Could you check a few things on this model? Use its own coordinates, in mm. Face numbers are marked on the shaded views. Coordinates: 2 decimals unless noted, no trailing zeros. Write each loop counter-clockwise with the first axis right and the second up, starting at its lowest first coordinate (ties: lowest second). Pieces come first, ordered by that corner, then holes. Notation, with made-up numbers: (-3, 67) - (51, 67) arc R19 ccw to (51, 84) - close; hole circle Ø5 at (35.5, 40.5). An arc over 180 degrees is marked (long way). Answer as a JSON object with one key per item and string values. Group by question number.
1) If we section it at B-B (y = -70): Write out the boundary of the cut face in (x, z).
2) If we section it at D-D (x = 70): Write out the boundary of the cut face in (y, z).
3) We'd pull the mould along Y, two halves only. Please class the marked faces 1, 2, 3 and 4: released by +Y, released by -Y, zero draft, split by the parting line, or undercut.
4) If we section it at A-A (y = -30): Write out the boundary of the cut face in (x, z).
5) Will these pins go through, and if not, where does the flat tip stop? pin 1 Ø5 at (x, y) = (30, -30) entering from -Z; pin 2 Ø2.5 at (x, z) = (22, 9.5) entering from -Y; pin 3 Ø4 at (y, z) = (-14.5, 9) entering from +X; pin 4 Ø24 at (x, y) = (38, -52.5) entering from +Z.
6) Please list where these lines run through material, in increasing order: line 1 along X through (y, z) = (-13, 10); line 2 along Y through (x, z) = (30, 1.85); line 3 along X through (y, z) = (-51, 3).
7) If we section it at C-C (z = 10): Write out the boundary of the cut face in (x, y).
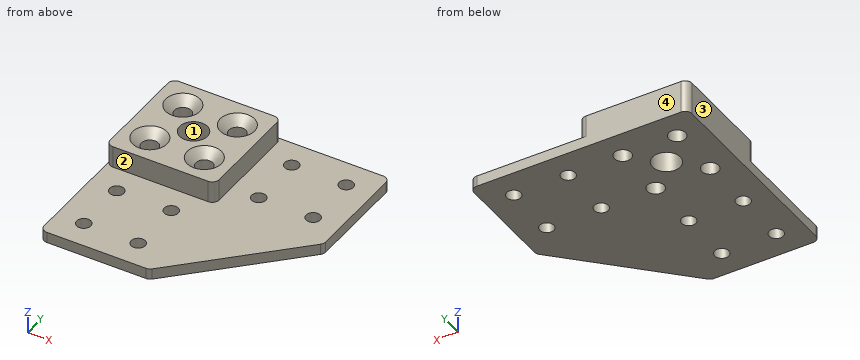
```python
from build123d import *

# Parameters (mm, degrees)
EXTRUDE_1_DEPTH             = 4
SKETCH_2_W                  = 40
SKETCH_2_H                  = 40
EXTRUDE_2_DEPTH             = 8
HOLE_WIZARD_M61_D           = 6.2
HOLE_WIZARD_M61_CSINK_D     = 12.6
HOLE_WIZARD_M61_CSINK_ANGLE = 90
SKETCH_5_R                  = 5.1
CUT_EXTRUDE_1_DEPTH         = 114.771701227
SKETCH_6_R                  = 2.6
CUT_EXTRUDE_2_DEPTH         = 114.41957503
FILLET_1_R                  = 2.5


with BuildPart() as part:
    # Эскиз1 → Бобышка-Вытянуть1 (new body)
    with BuildSketch(Plane.XY):
        Polygon((0, 0), (80, 0), (80, -40), (40, -80), (0, -80), align=None)
    extrude(amount=EXTRUDE_1_DEPTH)

    # Эскиз2 → Бобышка-Вытянуть2 (add)
    with BuildSketch(Plane.XY.offset(4)):
        with Locations((20, -20)):
            Rectangle(SKETCH_2_W, SKETCH_2_H)
    extrude(amount=EXTRUDE_2_DEPTH)

    # Зенковка для винта с полупотайной головкой M61 (through all)
    with Locations(Plane(origin=(10, -30, 12), x_dir=(1, 0, 0), z_dir=(0, 0, 1))):
        with Locations((0, 0), (0, 20), (20, 20), (20, 0)):
            CounterSinkHole(HOLE_WIZARD_M61_D / 2, HOLE_WIZARD_M61_CSINK_D / 2, counter_sink_angle=HOLE_WIZARD_M61_CSINK_ANGLE)

    # Эскиз5 → Вырез-Вытянуть1 (cut, through all)
    with BuildSketch(Plane.XY.offset(12)):
        with Locations((20, -20)):
            Circle(SKETCH_5_R)
    extrude(amount=-CUT_EXTRUDE_1_DEPTH, mode=Mode.SUBTRACT)

    # Эскиз6 → Вырез-Вытянуть2 (cut, through all)
    with BuildSketch(Plane.XY.offset(4)):
        with Locations((10, -50)):
            Circle(SKETCH_6_R)
        with Locations((30, -50)):
            Circle(SKETCH_6_R)
        with Locations((30, -70)):
            Circle(SKETCH_6_R)
        with Locations((10, -70)):
            Circle(SKETCH_6_R)
        with Locations(Location((70, -10, 0), (0, 0, 180))):
            Circle(SKETCH_6_R)
        with Locations(Location((70, -30, 0), (0, 0, 180))):
            Circle(SKETCH_6_R)
        with Locations(Location((50, -30, 0), (0, 0, 180))):
            Circle(SKETCH_6_R)
        with Locations(Location((50, -10, 0), (0, 0, 180))):
            Circle(SKETCH_6_R)
    extrude(amount=-CUT_EXTRUDE_2_DEPTH, mode=Mode.SUBTRACT)

    # Скругление1
    fillet_1_edges = [part.edges().sort_by_distance(p)[0] for p in [
        (0, -40, 8),
        (40, -40, 8),
        (40, 0, 8),
        (0, 0, 6),
        (80, 0, 2),
        (80, -40, 2),
        (40, -80, 2),
        (0, -80, 2),
    ]]
    fillet(fillet_1_edges, radius=FILLET_1_R)


solid = part.part
```
Here are the results:
{
 "1": {"outline": "(0, 0) - (7.4, 0) - (7.4, 4) - (0, 4) - close; (12.6, 0) - (27.4, 0) - (27.4, 4) - (12.6, 4) - close; (32.6, 0) - (50, 0) - (50, 4) - (32.6, 4) - close"},
 "2": {"outline": "(-50, 0) - (-32.6, 0) - (-32.6, 4) - (-50, 4) - close; (-27.4, 0) - (-12.6, 0) - (-12.6, 4) - (-27.4, 4) - close; (-7.4, 0) - (0, 0) - (0, 4) - (-7.4, 4) - close"},
 "3": {"face 1": "undercut", "face 2": "released by -Y", "face 3": "zero draft", "face 4": "released by +Y"},
 "4": {"outline": "(0, 0) - (6.9, 0) - (6.9, 8.8) - (3.7, 12) - (0, 12) - close; (13.1, 0) - (26.9, 0) - (26.9, 8.8) - (23.7, 12) - (16.3, 12) - (13.1, 8.8) - close; (33.1, 0) - (47.4, 0) - (47.4, 4) - (40, 4) - (40, 12) - (36.3, 12) - (33.1, 8.8) - close; (52.6, 0) - (67.4, 0) - (67.4, 4) - (52.6, 4) - close; (72.6, 0) - (80, 0) - (80, 4) - (72.6, 4) - close"},
 "5": {"pin 1": "passes through", "pin 2": "stops at y = -40", "pin 3": "stops at x = 40", "pin 4": "stops at z = 4"},
 "6": {"line 1": "x = 0 to 6.92, 13.08 to 26.92, 33.08 to 40", "line 2": "y = -80 to -72.6, -67.4 to -52.6, -47.4 to -33.1, -26.9 to -13.1, -6.9 to 0", "line 3": "x = 0 to 7.6, 12.4 to 27.6, 32.4 to 69"},
 "7": {"outline": "(0, -37.5) arc R2.5 ccw to (2.5, -40) - (37.5, -40) arc R2.5 ccw to (40, -37.5) - (40, -2.5) arc R2.5 ccw to (37.5, 0) - (2.5, 0) arc R2.5 ccw to (0, -2.5) - close; hole circle Ø8.6 at (10, -30); hole circle Ø8.6 at (10, -10); hole circle Ø10.2 at (20, -20); hole circle Ø8.6 at (30, -30); hole circle Ø8.6 at (30, -10)"}
}
